```python
from build123d import *

# Parameters (mm, degrees)
AUFSATZ_LINEAR_AUSTRAGEN1_DEPTH      = 15
SKIZZE2_W                            = 50
SKIZZE2_H                            = 40
AUFSATZ_LINEAR_AUSTRAGEN2_DEPTH      = 5
AUFSATZ_LINEAR_AUSTRAGEN2_DEPTH_BACK = 1
SKIZZE3_W                            = 23
SKIZZE3_H                            = 7
AUFSATZ_LINEAR_AUSTRAGEN3_DEPTH      = 5
SKIZZE4_W                            = 15
SKIZZE4_H                            = 15
AUFSATZ_LINEAR_AUSTRAGEN4_DEPTH      = 20


with BuildPart() as part:
    # Skizze1 → Aufsatz-Linear austragen1 (new body)
    with BuildSketch(Plane.XY):
        with BuildLine():
            Line((0, 0), (0, 70))
            Line((0, 70), (-12, 70))
            Line((-12, 70), (-12, 23.5))
            ThreePointArc((-12, 23.5), (-23.5, 12), (-35, 23.5))
            Line((-35, 23.5), (-35, 70))
            Line((-35, 70), (-47, 70))
            Line((-47, 70), (-47, 23.5))
            ThreePointArc((-47, 23.5), (-35.374342087, 3.220700209), (-12, 3.006098468))
            Line((-12, 3.006098468), (-12, 0))
            Line((-12, 0), (0, 0))
        make_face()
    extrude(amount=AUFSATZ_LINEAR_AUSTRAGEN1_DEPTH)

    # Skizze2 → Aufsatz-Linear austragen2 (add, two sides)
    with BuildSketch(Plane.XZ) as aufsatz_linear_austragen2_sk:
        with Locations((-23.5, 7.5)):
            Rectangle(SKIZZE2_W, SKIZZE2_H)
    extrude(amount=AUFSATZ_LINEAR_AUSTRAGEN2_DEPTH)
    extrude(aufsatz_linear_austragen2_sk.sketch, amount=-AUFSATZ_LINEAR_AUSTRAGEN2_DEPTH_BACK)

    # Skizze3 → Aufsatz-Linear austragen3 (add)
    with BuildSketch(Plane(origin=(0, 70, 0), x_dir=(1, 0, 0), z_dir=(0, 1, 0))):
        with Locations((-23.5, -7.5)):
            Rectangle(SKIZZE3_W, SKIZZE3_H)
    extrude(amount=-AUFSATZ_LINEAR_AUSTRAGEN3_DEPTH)

    # Skizze4 → Aufsatz-Linear austragen4 (add)
    with BuildSketch(Plane(origin=(0, 70, 0), x_dir=(1, 0, 0), z_dir=(0, 1, 0))):
        with Locations((-23.5, -7.5)):
            Rectangle(SKIZZE4_W, SKIZZE4_H)
    extrude(amount=AUFSATZ_LINEAR_AUSTRAGEN4_DEPTH)


solid = part.part
```
Model file for the job. Use its own axes, mm. A direction names the side the tool comes from. Coordinates: 2 decimals unless noted, no trailing zeros. Order: outer loops, then holes, each group sorted by start corner. A loop starts at its lowest first (then second) coordinate and runs counter-clockwise, first axis right, second up. Notation, with made-up numbers: (-28, -34) -> (22, -34) arc R20 cw to (22, -29) -> close; hole circle Ø3 at (13, 39). An arc over 180 degrees is marked (long way). Return JSON: item names as keys, results as strings.
Item 1: 3-axis set-ups, long thin cutter, end or side, ignore diameter. For faces 1 (the face through (-24, 70, 13)), 2 (the face through (0, 35, 7)), 3 (the face through (-24, 80, 0)), 4 (the face through (-31, 80, 8)): which of +Z, -Z, +X, -X, +Y, -Y reach the whole face in a straight line?
Model answer:
{"face 1": "+Z", "face 2": "+Z, -Z, +X, +Y", "face 3": "-Z, +X, -X, +Y", "face 4": "+Z, -Z, -X, +Y"}
Item 2: Slice it at D-D (z = -4). Write the cut outline in (x, y), then the cut area to 3 significant figures.
Model answer:
{"outline": "(-48.5, -5) -> (1.5, -5) -> (1.5, 1) -> (-48.5, 1) -> close", "area": "300 mm²"}
Item 3: Slice it at A-A (x = -23.5). Write the cut outline in (y, z), then the cut area to 3 significant figures.
Model answer:
{"outline": "(-5, -12.5) -> (1, -12.5) -> (1, 0) -> (12, 0) -> (12, 15) -> (1, 15) -> (1, 27.5) -> (-5, 27.5) -> close; (65, 4) -> (70, 4) -> (70, 0) -> (90, 0) -> (90, 15) -> (70, 15) -> (70, 11) -> (65, 11) -> close", "area": "740 mm²"}
Item 4: Slice it at B-B (y = 41). Write the cut outline in (x, z), then the cut area to 3 significant figures.
Model answer:
{"outline": "(-47, 0) -> (-35, 0) -> (-35, 15) -> (-47, 15) -> close; (-12, 0) -> (0, 0) -> (0, 15) -> (-12, 15) -> close", "area": "360 mm²"}
Item 5: Mould opens along X. For faces 5 (the face through (-14.34, 1.86, 7.4)), 6 (the face through (-24, 80, 15)), 7 (the face through (1.5, -2, 7)) say: pulls with the +X half, pulls with the -X half, needs draft (parallel to the pull), parting line crosses it, or undercut.
Model answer:
{"face 5": "undercut", "face 6": "needs draft", "face 7": "pulls with the +X half"}
Item 6: Wall check: line 1 along X through (y, z) = (37, 8.5); line 2 along Z through (x, y) = (-42, 56.5); line 3 along Y through (x, z) = (-36, -4.5). Give the ranges that are in metal, low to high. Write a range as from..to.
Model answer:
{"line 1": "x = -47..-35, -12..0", "line 2": "z = 0..15", "line 3": "y = -5..1"}
Item 7: Slice it at C-C (x = -4). Write the cut outline in (y, z).
Model answer:
{"outline": "(-5, -12.5) -> (1, -12.5) -> (1, 0) -> (70, 0) -> (70, 15) -> (1, 15) -> (1, 27.5) -> (-5, 27.5) -> close"}
Item 8: Pin check, flat tips, straight feed: P1, Ø3, axis at x = -11, y = 10.5, coming from the -Z side; P2, Ø1, axis at y = 67, z = 13, coming from the +X side; P3, Ø16.5, axis at y = 77.5, z = 5.5, coming from the -X side. Stop position of each tip, or through.
Model answer:
{"P1": "stops at z = 0", "P2": "stops at x = 0", "P3": "stops at x = -47"}
